Input: part model. Units: mm. Frame: model coordinates. A direction names the side the tool comes from. Give positions to 0.01 mm unless a question says otherwise; leave off trailing zeros. Loops run counter-clockwise (first coordinate to the right, second up) from the corner with the lowest first, then second, coordinate; pieces in that order, holes last. Notation, with made-up numbers: (82.25, 49.5) -> (98.25, 49.5) arc R17 ccw to (98.25, 67.5) -> close; hole circle Ø1 at (-9.5, 72.25). An arc over 180 degrees is marked (long way). One line per question, with ' | ' between items.
Solid Edge part; units mm, degrees
sketch "Sketch1" plane through (0, 0, 0) normal (0, -1, 0) x (1, 0, 0)
  circle A0 centre (0, 0) radius 67
extrude "Protrusion1" add sketch "Sketch1" against normal blind 22
sketch "Sketch2" plane through (0, 0, 0) normal (1, 0, 0) x (0, 1, 0)
  line L0 (8.56, 67) -> (8.56, 45.9948)
  arc A0 (8.56, 45.9948) -> (11.5548, 43) centre (11.5548, 45.9948) ccw
  line L1 (22, 43) -> (11.5548, 43)
  line L2 (22, 67) -> (22, 43)
  line L3 (8.56, 67) -> (22, 67)
revolve "RevolvedCutout1" cut sketch "Sketch2" angle 360 about axis through (0, 0, 0) along (0, 1, 0)
sketch "Sketch3" plane through (0, 0, 0) normal (0, -1, 0) x (1, 0, 0)
  circle A0 centre (0, 0) radius 12.5
extrude "ExtrudedCutout_1" cut sketch "Sketch3" against normal blind 22
1. Section query B-B (z = 0). Output: boundary loops of the cut face in (x, y).
Determined:
outline: (-67, 0) -> (-12.5, 0) -> (-12.5, 22) -> (-43, 22) -> (-43, 11.55) arc R2.99 cw to (-45.99, 8.56) -> (-67, 8.56) -> close; (12.5, 0) -> (67, 0) -> (67, 8.56) -> (45.99, 8.56) arc R2.99 cw to (43, 11.55) -> (43, 22) -> (12.5, 22) -> close
2. Section query A-A (x = 0). Output: boundary loops of the cut face in (y, z).
Determined:
outline: (0, -67) -> (8.56, -67) -> (8.56, -45.99) arc R2.99 cw to (11.55, -43) -> (22, -43) -> (22, -12.5) -> (0, -12.5) -> close; (0, 12.5) -> (22, 12.5) -> (22, 43) -> (11.55, 43) arc R2.99 cw to (8.56, 45.99) -> (8.56, 67) -> (0, 67) -> close
3. Section query D-D (y = 19.25). Output: boundary loops of the cut face in (x, z), then the cut area to 3 significant figures.
Determined:
outline: circle Ø86 at (0, 0); hole circle Ø25 at (0, 0) | area: 5,320 mm2
4. Section query C-C (y = 4.25). Output: boundary loops of the cut face in (x, z).
Determined:
outline: circle Ø134 at (0, 0); hole circle Ø25 at (0, 0)
5. Pin query (flat end, axial travel): P1, Ø8, axis at x = 52.5, y = 9.5, coming from the -Z side; P2, Ø1.5, axis at y = 5.5, z = -2, coming from the -X side; P3, Ø1, axis at x = 33, y = 12, coming from the -Z side. Return the tip coordinate at first contact, or that it passes through.
Determined:
P1: stops at z = -46.11 | P2: stops at x = -66.99 | P3: stops at z = -28.16
6. Reachability of faces 4 (the cylindrical face through (-42.634, 16.704, -5.598)), 5 (the flat face through (-9, 22, -9)) from +Z, -Z, +X, -X, +Y, -Y: full face, straight path, thin tool, end or side. Return the list, or none.
Determined:
face 4: +Y | face 5: +Z, -Z, +X, -X, +Y
7. Ray query, line 1 along Y through (x, z) = (-49, 37.5); line 2 along X through (y, z) = (9, -10.5); line 3 along Z through (x, y) = (-42.5, 1). Return the intervals inside material, ascending. Write a range as from..to.
Determined:
line 1: y = 0..8.56 | line 2: x = -43.17..-6.78, 6.78..43.17 | line 3: z = -51.8..51.8
8. Pull-direction query (X, two-part tool) for faces 1 (the cylindrical face through (-14.524, 4.22, -65.407)), 2 (the cylindrical face through (11.923, 10.846, 3.755)), 3 (the flat face through (-14, 0, 1)); classes: pulls with the +X half, pulls with the -X half, needs draft (parallel to the pull), parting line crosses it, or undercut.
Determined:
face 1: parting line crosses it | face 2: undercut | face 3: needs draft
